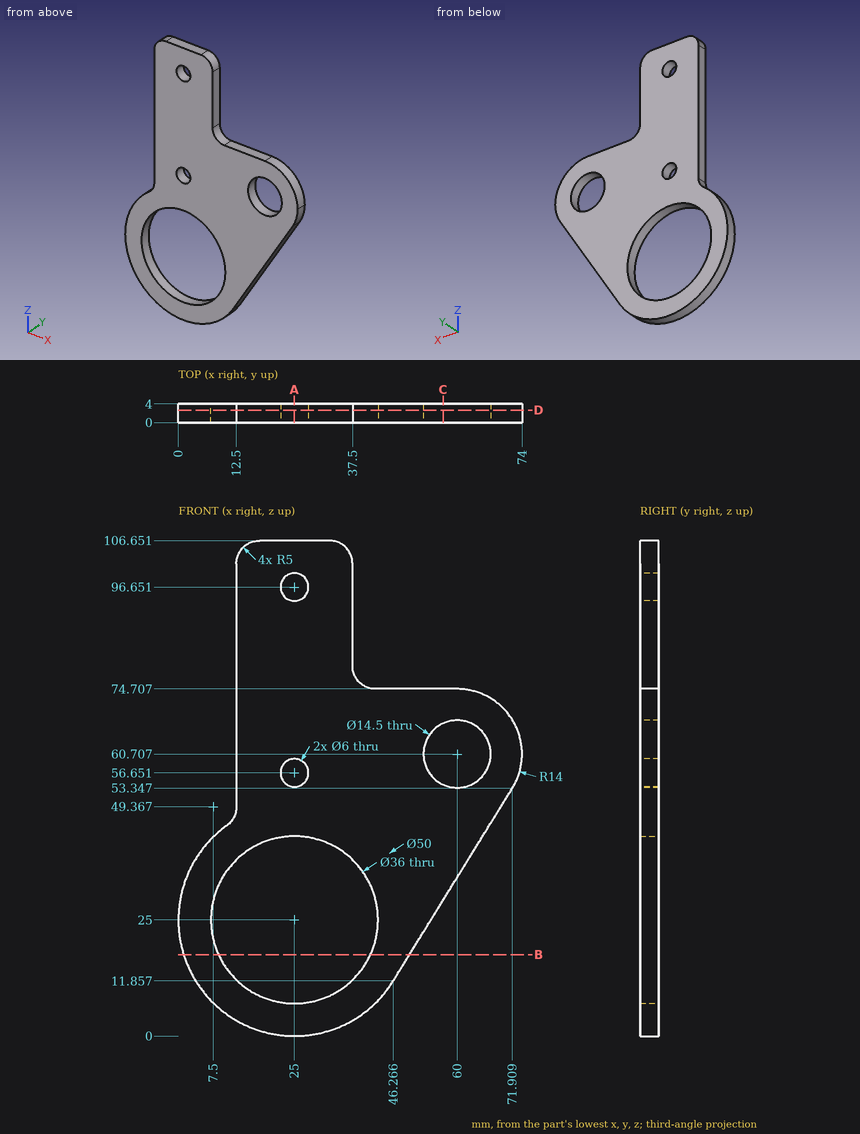
Here's the drawing with two shaded views (mm, measured from the low corner). I have some questions. Round coordinates to 2 decimals unless told otherwise and drop trailing zeros. Loops run counter-clockwise (first coordinate to the right, second up) from the corner with the lowest first, then second, coordinate; pieces in that order, holes last.
Item 1: Suppose I cut it at B-B, the plane z = 17.5. Write out the boundary of the cut face in (x, y) (1 decimal).
Item 2: Please list where these lines run through material, in increasing order: L1, parallel to Z at x = 25, y = 1.2; L2, parallel to Z at x = 60, y = 1.6 (1 decimal); L3, parallel to X at y = 0.6, z = 97.5.
Item 3: Suppose I cut it at A-A, the plane x = 25. Write out the boundary of the cut face in (y, z).
Item 4: Will these pins go through, and if not, where does the flat tip stop? pin 1 Ø1.2 at (y, z) = (1, 65) entering from -X; pin 2 Ø2 at (y, z) = (1.5, 36.5) entering from -X; pin 3 Ø1 at (y, z) = (2, 42) entering from +X (1 decimal); pin 4 Ø11.5 at (x, z) = (60, 60.71) entering from -Y.
Item 5: Suppose I cut it at D-D, the plane y = 2.7. State how many separate pieces and enclosed holes the cut face has, then the cut area to 3 significant figures.
Item 6: Suppose I cut it at C-C, the plane x = 57. Write out the boundary of the cut face in (y, z).
Reported:
1. outline: (1.2, 0) - (8.6, 0) - (8.6, 4) - (1.2, 4) - close; (41.4, 0) - (49.8, 0) - (49.8, 4) - (41.4, 4) - close
2. L1: z = 0 to 7, 43 to 53.65, 59.65 to 93.65, 99.65 to 106.65
2. L2: z = 34.1 to 53.5, 68 to 74.7
2. L3: x = 12.5 to 22.12, 27.88 to 37.5
3. outline: (0, 0) - (4, 0) - (4, 7) - (0, 7) - close; (0, 43) - (4, 43) - (4, 53.65) - (0, 53.65) - close; (0, 59.65) - (4, 59.65) - (4, 93.65) - (0, 93.65) - close; (0, 99.65) - (4, 99.65) - (4, 106.65) - (0, 106.65) - close
4. pin 1: stops at x = 12.5
4. pin 2: stops at x = 2.31
4. pin 3: stops at x = 65.2
4. pin 4: passes through
5. separate pieces: 1
5. enclosed holes: 4
5. area: 3,450 mm2
6. outline: (0, 29.22) - (4, 29.22) - (4, 54.11) - (0, 54.11) - close; (0, 67.31) - (4, 67.31) - (4, 74.71) - (0, 74.71) - close
